```python
from build123d import *

# Parameters (mm, degrees)
SKETCH_1_W            = 60
SKETCH_1_H            = 75
EXTRUDE_1_DEPTH       = 55
CUT_EXTRUDE_2_DEPTH   = 63
CUT_EXTRUDE_3_DEPTH   = 63
CUT_EXTRUDE_4_DEPTH   = 63
CUT_EXTRUDE_5_DEPTH   = 73
CUT_EXTRUDE_6_DEPTH   = 32
CUT_EXTRUDE_7_DEPTH   = 32
EXTRUDE_2_DEPTH       = 2
SKETCH_10_W           = 1
SKETCH_10_H           = 20
EXTRUDE_3_DEPTH       = 20
FILLET_1_R            = 5
HOLE_WIZARD_M51_D     = 4.2
HOLE_WIZARD_M51_DEPTH = 38.5
HOLE_WIZARD_M51_TIP   = 1.2618073


with BuildPart() as part:
    # Эскиз1 → Бобышка-Вытянуть1 (new body)
    with BuildSketch(Plane.XY):
        with Locations((30, 37.5)):
            Rectangle(SKETCH_1_W, SKETCH_1_H)
    extrude(amount=EXTRUDE_1_DEPTH)

    # Эскиз3 → Вырез-Вытянуть2 (cut)
    with BuildSketch(Plane(origin=(60, 0, 0), x_dir=(0, 0, -1), z_dir=(1, 0, 0))):
        Polygon((0, 0), (0, 10), (-20, 0), align=None)
        Polygon((0, 75), (0, 70), (-25, 75), align=None)
    extrude(amount=-CUT_EXTRUDE_2_DEPTH, mode=Mode.SUBTRACT)

    # Эскиз4 → Вырез-Вытянуть3 (cut)
    with BuildSketch(Plane(origin=(0, 0, 0), x_dir=(-1, 0, 0), z_dir=(0, 0, -1))):
        Polygon((-60, 0), (-60, 10), (-43, 0), align=None)
    extrude(amount=-CUT_EXTRUDE_3_DEPTH, mode=Mode.SUBTRACT)

    # Эскиз5 → Вырез-Вытянуть4 (cut)
    with BuildSketch(Plane(origin=(0, 0, 0), x_dir=(-1, 0, 0), z_dir=(0, 0, -1))):
        Polygon((-60, 75), (-60, 65), (-50, 75), align=None)
        Polygon((-10, 75), (0, 65), (0, 75), align=None)
    extrude(amount=-CUT_EXTRUDE_4_DEPTH, mode=Mode.SUBTRACT)

    # Эскиз6 → Вырез-Вытянуть5 (cut)
    with BuildSketch(Plane(origin=(0, 75, 0), x_dir=(1, 0, 0), z_dir=(0, 1, 0))):
        with BuildLine():
            Line((30.000000357, 0), (0, 0))
            Line((0, 0), (0, -4.606079858))
            ThreePointArc((0, -4.606079858), (14.824230248, -1.158227391), (30.000000357, 0))
        make_face()
        with BuildLine():
            Line((60, 0), (30.000000357, 0))
            ThreePointArc((30.000000357, 0), (45.175770105, -1.158227445), (60, -4.606079858))
            Line((60, -4.606079858), (60, 0))
        make_face()
    extrude(amount=-CUT_EXTRUDE_5_DEPTH, mode=Mode.SUBTRACT)

    # Эскиз7 → Вырез-Вытянуть6 (cut)
    with BuildSketch(Plane.XY.offset(55)):
        Polygon((58, 64.171572875), (49.171572875, 73), (10.828427125, 73), (2, 64.171572875), (2, 2), (42.455383415, 2), (58, 11.143892109), align=None)
    extrude(amount=-CUT_EXTRUDE_6_DEPTH, mode=Mode.SUBTRACT)

    # Эскиз8 → Вырез-Вытянуть7 (cut)
    with BuildSketch(Plane(origin=(60, 0, 0), x_dir=(0, 0, -1), z_dir=(1, 0, 0))):
        Polygon((-55, 18.854810441), (-55, 53.166098562), (-41, 51.5), (-41, 20), align=None)
    extrude(amount=-CUT_EXTRUDE_7_DEPTH, mode=Mode.SUBTRACT)

    # Эскиз9 → Бобышка-Вытянуть2 (add)
    with BuildSketch(Plane.ZY.offset(-58)):
        Polygon((55, 53.166098562), (55, 18.854810441), (55, 12.004066058), (30, 12.004066058), (30, 58.166098562), (55, 58.166098562), align=None)
    extrude(amount=EXTRUDE_2_DEPTH)

    # Эскиз10 → Бобышка-Вытянуть3 (add)
    with BuildSketch(Plane(origin=(58, 0, 0), x_dir=(0, 0, -1), z_dir=(1, 0, 0))):
        with Locations((-50.5, 35.75)):
            Rectangle(SKETCH_10_W, SKETCH_10_H)
    extrude(amount=EXTRUDE_3_DEPTH)

    # Скругление1
    fillet_1_edges = [part.edges().sort_by_distance(p)[0] for p in [
        (78, 45.75, 50.5),
        (78, 25.75, 50.5),
    ]]
    fillet(fillet_1_edges, radius=FILLET_1_R)

    # Отверстие обработанное метчиком M51
    with Locations(Plane(origin=(0, 0, 50), x_dir=(-1, 0, 0), z_dir=(0, 0, -1))):
        with Locations((-70.936057607, 36.012290947)):
            Hole(HOLE_WIZARD_M51_D / 2, depth=HOLE_WIZARD_M51_DEPTH)
            with Locations((0, 0, -(HOLE_WIZARD_M51_DEPTH + HOLE_WIZARD_M51_TIP / 2))):  # 118° drill point
                Cone(0, HOLE_WIZARD_M51_D / 2, HOLE_WIZARD_M51_TIP, mode=Mode.SUBTRACT)


solid = part.part
```
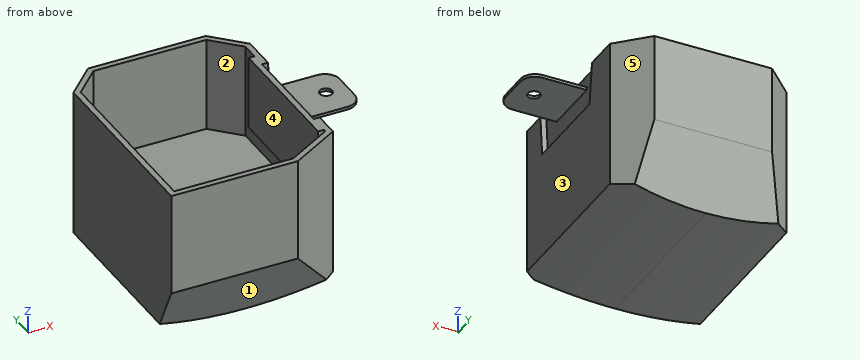
The model under review builds one solid part; all positions refer to its coordinate system, in mm. Face numbers are marked on the shaded views. A direction names the side the tool comes from. Round coordinates to 2 decimals unless told otherwise and drop trailing zeros. Loops run counter-clockwise (first coordinate to the right, second up) from the corner with the lowest first, then second, coordinate; pieces in that order, holes last. Notation, with made-up numbers: M 1,84 L 20,84 A32 cw 20,113 Z; hole C 86,-9.75 d5. An arc over 180 degrees is marked long. Put each result on its own line as item: value.
Q1. Mouldability with a two-part tool opening along Y and no side actions: class the marked faces 3, 4 and 5 as released by +Y, released by -Y, zero draft, split by the parting line, or undercut.
Result set:
face 3: zero draft
face 4: undercut
face 5: released by +Y
Q2. Consider section A-A, the plane z = 40. Give the boundary of the cut face in (x, y), then the cut area to 3 significant figures.
Result set:
outline: M 0,0 L 43,0 L 60,10 L 60,65 L 50,75 L 10,75 L 0,65 Z; hole M 2,2 L 42.46,2 L 58,11.14 L 58,12 L 56,12 L 56,58.17 L 58,58.17 L 58,64.17 L 49.17,73 L 10.83,73 L 2,64.17 Z
area: 580 mm²
Q3. To check wall thickness, follow L1, parallel to Y at x = 18.5, z = 42.5; L2, parallel to X at y = 47, z = 35; L3, parallel to X at y = 26, z = 46.5. State the ranges of each line that lie inside material, in increasing order.
Result set:
L1: y = 0 to 2, 73 to 75
L2: x = 0 to 2, 56 to 60
L3: x = 0 to 2, 56 to 58
Q4. Consider section C-C, the plane y = 37. Give the boundary of the cut face in (x, z), then the cut area to 3 significant figures.
Result set:
outline: M 0,4.61 A100 ccw 60,4.61 L 60,41 L 58,41 L 58,50 L 69.08,50 L 69.08,51 L 58,51 L 58,55 L 56,55 L 56,30 L 58,30 L 58,23 L 2,23 L 2,55 L 0,55 Z; M 72.79,50 L 78,50 L 78,51 L 72.79,51 Z
area: 1,460 mm²
Q5. Consider section D-D, the plane x = 41. Give the boundary of the cut face in (y, z).
Result set:
outline: M 0,20 L 9.7,0.61 L 70.12,0.61 L 75,25 L 75,55 L 73,55 L 73,23 L 2,23 L 2,55 L 0,55 Z
Q6. Machinability: for the marked faces 1 and 2, which of the approach directions +Z, -Z, +X, -X, +Y, -Y give a long, thin tool a straight path to every point of the face, cutting with its end or side? Answer none if there is none.
Result set:
face 1: -Z, +X, -X, -Y
face 2: +Z
Q7. For pin 1 (4 mm diameter, centred on x = 70.94, y = 36.01, fed in from +Z); pin 2 (0.8 mm diameter, centred on x = 66.5, z = 50.5, fed in from +Y); pin 3 (5 mm diameter, centred on x = 45.5, y = 37, fed in from -Z); pin 4 (5 mm diameter, centred on x = 54.5, z = 15, fed in from -Y), all flat-tipped, find the tip position at first contact; note any pin that passes through.
Result set:
pin 1: passes through
pin 2: stops at y = 45.75
pin 3: stops at z = 0.85
pin 4: stops at y = 5.29
Q8. Consider section B-B, the plane z = 10. Give the boundary of the cut face in (x, y).
Result set:
outline: M 0,5 L 51.5,5 L 60,10 L 60,65 L 53,72 L 7,72 L 0,65 Z
